Here's how the part is built. I have some questions about the finished solid (model axes, mm). Coordinates: 2 decimals unless noted, no trailing zeros. Order: outer loops, then holes, each group sorted by start corner. A loop starts at its lowest first (then second) coordinate and runs counter-clockwise, first axis right, second up. Notation, with made-up numbers: (-15, -31.5) -> (42, -31.5) arc R18 cw to (42, -7.5) -> close; hole circle Ø1 at (-16, 47). An arc over 180 degrees is marked (long way). One line per item, written item: value. Start each with the question number.
```python
from build123d import *

# Parameters (mm, degrees)
SKETCH1_W           = 1.6637
SKETCH1_H           = 1.1049
BOSS_EXTRUDE1_DEPTH = 101.6
CUT_EXTRUDE1_REACH  = 103.652
SKETCH2_R           = 0.889


with BuildPart() as part:
    # Sketch1 → Boss-Extrude1 (new body)
    with BuildSketch(Plane(origin=(0, 0, 0), x_dir=(1, 0, 0), z_dir=(0, 1, 0))):
        with Locations((-0.83185, 1.60655)):
            Rectangle(SKETCH1_W, SKETCH1_H)
        with Locations((0.83185, 1.60655)):
            Rectangle(SKETCH1_W, SKETCH1_H)
        Polygon((0, 1.0541), (0, 0), (2.4384, 0), (2.4384, 1.0541), (1.6637, 1.0541), align=None)
        Polygon((-2.4384, 0), (0, 0), (0, 1.0541), (-1.6637, 1.0541), (-2.4384, 1.0541), align=None)
    extrude(amount=BOSS_EXTRUDE1_DEPTH)

    # Sketch2 → Cut-Extrude1 (cut, up to next)
    with BuildSketch(Plane(origin=(0, 0, -2.159), x_dir=(-1, 0, 0), z_dir=(0, 0, -1)), mode=Mode.PRIVATE) as cut_extrude1_sk1:
        with Locations((0, 6.35)):
            Circle(SKETCH2_R)
    cut_extrude1_tool1 = extrude(cut_extrude1_sk1.sketch, amount=-CUT_EXTRUDE1_REACH, mode=Mode.PRIVATE) & part.part
    # Sketch2 → Cut-Extrude1 (cut, up to next)
    with BuildSketch(Plane(origin=(0, 0, -2.159), x_dir=(-1, 0, 0), z_dir=(0, 0, -1)), mode=Mode.PRIVATE) as cut_extrude1_sk2:
        with Locations((0, 19.05)):
            Circle(SKETCH2_R)
    cut_extrude1_tool2 = extrude(cut_extrude1_sk2.sketch, amount=-CUT_EXTRUDE1_REACH, mode=Mode.PRIVATE) & part.part
    # Sketch2 → Cut-Extrude1 (cut, up to next)
    with BuildSketch(Plane(origin=(0, 0, -2.159), x_dir=(-1, 0, 0), z_dir=(0, 0, -1)), mode=Mode.PRIVATE) as cut_extrude1_sk3:
        with Locations((0, 31.75)):
            Circle(SKETCH2_R)
    cut_extrude1_tool3 = extrude(cut_extrude1_sk3.sketch, amount=-CUT_EXTRUDE1_REACH, mode=Mode.PRIVATE) & part.part
    # Sketch2 → Cut-Extrude1 (cut, up to next)
    with BuildSketch(Plane(origin=(0, 0, -2.159), x_dir=(-1, 0, 0), z_dir=(0, 0, -1)), mode=Mode.PRIVATE) as cut_extrude1_sk4:
        with Locations((0, 44.45)):
            Circle(SKETCH2_R)
    cut_extrude1_tool4 = extrude(cut_extrude1_sk4.sketch, amount=-CUT_EXTRUDE1_REACH, mode=Mode.PRIVATE) & part.part
    # Sketch2 → Cut-Extrude1 (cut, up to next)
    with BuildSketch(Plane(origin=(0, 0, -2.159), x_dir=(-1, 0, 0), z_dir=(0, 0, -1)), mode=Mode.PRIVATE) as cut_extrude1_sk5:
        with Locations((0, 57.15)):
            Circle(SKETCH2_R)
    cut_extrude1_tool5 = extrude(cut_extrude1_sk5.sketch, amount=-CUT_EXTRUDE1_REACH, mode=Mode.PRIVATE) & part.part
    # Sketch2 → Cut-Extrude1 (cut, up to next)
    with BuildSketch(Plane(origin=(0, 0, -2.159), x_dir=(-1, 0, 0), z_dir=(0, 0, -1)), mode=Mode.PRIVATE) as cut_extrude1_sk6:
        with Locations((0, 69.85)):
            Circle(SKETCH2_R)
    cut_extrude1_tool6 = extrude(cut_extrude1_sk6.sketch, amount=-CUT_EXTRUDE1_REACH, mode=Mode.PRIVATE) & part.part
    # Sketch2 → Cut-Extrude1 (cut, up to next)
    with BuildSketch(Plane(origin=(0, 0, -2.159), x_dir=(-1, 0, 0), z_dir=(0, 0, -1)), mode=Mode.PRIVATE) as cut_extrude1_sk7:
        with Locations((0, 82.55)):
            Circle(SKETCH2_R)
    cut_extrude1_tool7 = extrude(cut_extrude1_sk7.sketch, amount=-CUT_EXTRUDE1_REACH, mode=Mode.PRIVATE) & part.part
    # Sketch2 → Cut-Extrude1 (cut, up to next)
    with BuildSketch(Plane(origin=(0, 0, -2.159), x_dir=(-1, 0, 0), z_dir=(0, 0, -1)), mode=Mode.PRIVATE) as cut_extrude1_sk8:
        with Locations((0, 95.25)):
            Circle(SKETCH2_R)
    cut_extrude1_tool8 = extrude(cut_extrude1_sk8.sketch, amount=-CUT_EXTRUDE1_REACH, mode=Mode.PRIVATE) & part.part
    add(cut_extrude1_tool1.solids().sort_by_distance((0, 6.35, -2.159))[0], mode=Mode.SUBTRACT)
    add(cut_extrude1_tool2.solids().sort_by_distance((0, 19.05, -2.159))[0], mode=Mode.SUBTRACT)
    add(cut_extrude1_tool3.solids().sort_by_distance((0, 31.75, -2.159))[0], mode=Mode.SUBTRACT)
    add(cut_extrude1_tool4.solids().sort_by_distance((0, 44.45, -2.159))[0], mode=Mode.SUBTRACT)
    add(cut_extrude1_tool5.solids().sort_by_distance((0, 57.15, -2.159))[0], mode=Mode.SUBTRACT)
    add(cut_extrude1_tool6.solids().sort_by_distance((0, 69.85, -2.159))[0], mode=Mode.SUBTRACT)
    add(cut_extrude1_tool7.solids().sort_by_distance((0, 82.55, -2.159))[0], mode=Mode.SUBTRACT)
    add(cut_extrude1_tool8.solids().sort_by_distance((0, 95.25, -2.159))[0], mode=Mode.SUBTRACT)


solid = part.part
```
Q1. For P1, Ø1.6, axis at x = 0, y = 31.75, coming from the -Z side; P2, Ø2.5, axis at x = 0, y = 95.25, coming from the +Z side, each with a flat end and sliding along its axis, tell me the tip position at first contact or that it passes through.
Q2. Imagine slicing it at B-B (z = -1.8). Count the separate pieces of the cut face and the enclosed holes in it, plus the area to 3 significant figures.
Q3. If we mould it in two halves opening along Y, with no side actions, what happens to faces 1 (the face through (0, 101.6, -1)), 2 (the face through (0.12, 7.23, -1.09)), 3 (the face through (0, 50, -2.159))? For each: +Y half, -Y half, draft (parallel to the pull), parting line (faces both ways), or undercut.
Q4. I need wall thicknesses on line 1 (X direction, y = 57.15, z = -0.85); line 2 (X direction, y = 42, z = -1.4); line 3 (Z direction, x = -2.1, y = 79.5). Which ranges of each line are inside material? Lowest first, please.
Q5. Imagine slicing it at C-C (y = 80.5). Write out the boundary of the cut face in (x, z).
Q6. Imagine slicing it at A-A (y = 69.85). Write out the boundary of the cut face in (x, z).
Completed:
1. P1: passes through
1. P2: stops at z = 0
2. separate pieces: 1
2. enclosed holes: 8
2. area: 318 mm2
3. face 1: +Y half
3. face 2: undercut
3. face 3: draft
4. line 1: x = -2.44 to -0.89, 0.89 to 2.44
4. line 2: x = -1.66 to 1.66
4. line 3: z = -1.05 to 0
5. outline: (-2.44, -1.05) -> (-1.66, -1.05) -> (-1.66, -2.16) -> (1.66, -2.16) -> (1.66, -1.05) -> (2.44, -1.05) -> (2.44, 0) -> (-2.44, 0) -> close
6. outline: (-2.44, -1.05) -> (-1.66, -1.05) -> (-1.66, -2.16) -> (-0.89, -2.16) -> (-0.89, 0) -> (-2.44, 0) -> close; (0.89, -2.16) -> (1.66, -2.16) -> (1.66, -1.05) -> (2.44, -1.05) -> (2.44, 0) -> (0.89, 0) -> close
